Autodesk Inventor part; units mm, degrees
ref_plane "YZ Plane" through (0, 0, 0) normal (1, 0, 0) x (0, 1, 0)
ref_plane "XZ Plane" through (0, 0, 0) normal (0, 1, 0) x (-1, 0, 0)
ref_plane "XY Plane" through (0, 0, 0) normal (0, 0, 1) x (1, 0, 0)
sketch "Sketch1" plane through (0, 0, 0) normal (0, 1, 0) x (-1, 0, 0)
  line L0 (0, 0) -> (0, -15) construction
  line L1 (0, 0) -> (16, 0) construction
  arc A0 (-6, -15) -> (6, -15) centre (0, -15) ccw
  arc A1 (16, -6) -> (16, 6) centre (16, 0) ccw
  line L2 (-6, -15) -> (-6, -6)
  line L3 (0, -6) -> (-6, -6) construction
  line L4 (16, 6) -> (6, 6)
  line L5 (6, 6) -> (-6, 6) construction
  line L6 (-6, 6) -> (-6, -6) construction
  line L7 (16, -6) -> (6, -6)
  line L8 (6, -6) -> (0, -6) construction
  line L9 (6, -15) -> (6, -6)
  circle A2 centre (0, 0) radius 1.35
  line L10 (0, 0) -> (0, -12) construction
  line L11 (0, -12) -> (0, -15) construction
  line L12 (0, -15) -> (0, -18) construction
  line L13 (0, 0) -> (10, 0) construction
  line L14 (10, 0) -> (13, 0) construction
  line L15 (13, 0) -> (16, 0) construction
  line L16 (16, 0) -> (19, 0) construction
  circle A3 centre (19, 0) radius 0.75
  circle A4 centre (16, 0) radius 0.75
  circle A5 centre (13, 0) radius 0.75
  circle A6 centre (10, 0) radius 0.75
  circle A7 centre (0, -12) radius 0.75
  circle A8 centre (0, -15) radius 0.75
  circle A9 centre (0, -18) radius 0.75
  line L17 (6.8305, 0) -> (-5.2, 0)
  line L18 (0, -4.7373) -> (0, 4.2525)
  arc A10 (6, 15) -> (-6, 15) centre (0, 15) ccw
  line L19 (-6, 15) -> (-6, 6)
  line L20 (6, 15) -> (6, 6)
  circle A11 centre (0, 12) radius 0.75
  circle A12 centre (0, 15) radius 0.75
  circle A13 centre (0, 18) radius 0.75
  arc A14 (-16, 6) -> (-16, -6) centre (-16, 0) ccw
  line L21 (-16, 6) -> (-6, 6)
  line L22 (-16, -6) -> (-6, -6)
  circle A15 centre (-19, 0) radius 0.75
  circle A16 centre (-16, 0) radius 0.75
  circle A17 centre (-13, 0) radius 0.75
  circle A18 centre (-10, 0) radius 0.75
  dimension "d0" = 15
  dimension "d1" = 16
  dimension "d2" = 12
  dimension "d3" = 12
  dimension "d5" = 2.7
  dimension "d6" = 12
  dimension "d7" = 3
  dimension "d8" = 3
  dimension "d9" = 10
  dimension "d10" = 3
  dimension "d11" = 3
  dimension "d12" = 3
  dimension "d13" = 1.5
  dimension "d14" = 1.5
  dimension "d15" = 1.5
  dimension "d16" = 1.5
  dimension "d17" = 1.5
  dimension "d18" = 1.5
  dimension "d19" = 1.5
  dimension "d20" = 6
extrude "Extrusion1" add sketch "Sketch1" along normal blind 2.1
sketch "Sketch2" plane through (0, 2.1, 0) normal (0, 1, 0) x (1, 0, 0)
  circle A0 centre (0, 0) radius 3
  dimension "d23" = 6
extrude "Extrusion2" cut sketch "Sketch2" against normal blind 1.4
sketch "Sketch3" plane through (0, 0, 0) normal (0, -1, 0) x (1, 0, 0)
  circle A0 centre (0, 0) radius 1.35
  circle A1 centre (0, 0) radius 6
  dimension "d26" = 12
extrude "Extrusion3" add sketch "Sketch3" along normal blind 0.9
sketch "Sketch4" plane through (0, -0.9, 0) normal (0, -1, 0) x (1, 0, 0)
  circle A0 centre (0, 0) radius 1.35
  circle A1 centre (0, 0) radius 5
  dimension "d29" = 10
extrude "Extrusion4" add sketch "Sketch4" along normal blind 2.85
sketch "Sketch5" plane through (0, 0, 0) normal (0, -1, 0) x (1, 0, 0)
  line L0 (16, -6) -> (6, -6)
  arc A0 (-16, 6) -> (-16, -6) centre (-16, 0) ccw
  line L1 (16, -6) -> (-16, -6)
  line L2 (6, 6) -> (16, 6)
  line L3 (16, 6) -> (-16, 6)
  circle A1 centre (-16, 0) radius 0.75
  arc A2 (-16, 6) -> (-16, -6) centre (-16, 0) ccw
  circle A3 centre (16, 0) radius 0.75
  arc A4 (16, -6) -> (16, 6) centre (16, 0) ccw
  circle A5 centre (-10, 0) radius 0.75
  circle A6 centre (-10, 0) radius 0.75
  circle A7 centre (-13, 0) radius 0.75
  circle A8 centre (-13, 0) radius 0.75
  circle A9 centre (-19, 0) radius 0.75
  circle A10 centre (-19, 0) radius 0.75
  circle A11 centre (-16, 0) radius 0.75
  circle A12 centre (10, 0) radius 0.75
  circle A13 centre (10, 0) radius 0.75
  circle A14 centre (13, 0) radius 0.75
  circle A15 centre (13, 0) radius 0.75
  circle A16 centre (16, 0) radius 0.75
  circle A17 centre (19, 0) radius 0.75
  circle A18 centre (19, 0) radius 0.75
  point P0 (0, 0)
extrude "Extrusion5" add sketch "Sketch5" along normal blind 0.9
sketch "Sketch6" plane through (0, -0.9, 0) normal (0, -1, 0) x (1, 0, 0)
  circle A0 centre (0, 0) radius 1.35
  circle A1 centre (0, 0) radius 1.35
extrude "Extrusion6" cut sketch "Sketch6" against normal blind 0.9
sketch "Sketch7" plane through (0, -3.75, 0) normal (0, -1, 0) x (1, 0, 0)
  circle A0 centre (0, 0) radius 1.35
  circle A1 centre (0, 0) radius 2.75
  dimension "d36" = 5.5
extrude "Extrusion7" cut sketch "Sketch7" against normal blind 3 contours A0 | A1
properties part number "MMAE 232 CAD Assignment 2 Servo Horn 3-Nicholas Skiba"
Check sheet for the modelled part. Datum: model origin and axes. Units: mm. A direction names the side the tool comes from. Give positions to 0.01 mm unless a question says otherwise; leave off trailing zeros. Write each loop counter-clockwise with the first axis right and the second up, starting at its lowest first coordinate (ties: lowest second). Pieces come first, ordered by that corner, then holes. Notation, with made-up numbers: (24.5, -4.5) -> (64.5, -4.5) arc R18 ccw to (64.5, 30.5) -> close; hole circle Ø11 at (87.5, -29). An arc over 180 degrees is marked (long way). One line per item, written item: value. Start each with the question number.
Item 1: Section check A-A on x = 13. Record the cut outline in (y, z).
Item 2: Tool access check on faces 5 (the flat face through (0, 0, 14)), 6 (the flat face through (-6, 1, 11)), 7 (the flat face through (6, 1, -11)), 8 (the flat face through (6, 1, 11)), 9 (the flat face through (0, 0, -13)). Record the directions out of +Z, -Z, +X, -X, +Y, -Y that give a thin tool (end or side, any length) a straight path to the whole face; none if there is none.
Item 3: Gauge pin test, flat ends, axial feed: pin 1 (1 mm diameter, centred on x = -2.5, z = 1.5, fed in from +Y); pin 2 (1.7 mm diameter, centred on x = -16, z = 0, fed in from -Y); pin 3 (2.5 mm diameter, centred on x = -1.5, y = 1, fed in from +Z); pin 4 (1.5 mm diameter, centred on x = 4.5, z = -10, fed in from -Y). Record the tip position at first contact, or that the pin passes through.
Item 4: Material ranges on probe 1 along Z at (x, y) = (-13, -0.45); probe 2 along Z at (x, y) = (0, -0.5); probe 3 along Y at (x, z) = (19, -2), recorded low to high. Write a range as from..to.
Item 5: Section check B-B on z = 18. Record the cut outline in (x, y).
Item 6: Section check C-C on y = -3.2. Record the cut outline in (x, z).
Item 7: Draft check along Z on faces 1 (the cylindrical face through (0.098, 1.035, 11.256)), 2 (the cylindrical face through (22, 1, 0)), 3 (the cylindrical face through (0, 1, 21)), 4 (the cylindrical face through (-3, 1, 0)). Enter one of: +Z half, -Z half, draft (parallel to the pull), parting line (faces both ways), or undercut.
Item 8: Section check D-D on z = -3.5. Record the cut outline in (x, y).
Results list:
1. outline: (-0.9, -6) -> (2.1, -6) -> (2.1, -0.75) -> (-0.9, -0.75) -> close; (-0.9, 0.75) -> (2.1, 0.75) -> (2.1, 6) -> (-0.9, 6) -> close
2. face 5: +Z, +X, -X, -Y
2. face 6: +Z, -X, +Y, -Y
2. face 7: -Z, +X, +Y, -Y
2. face 8: +Z, +X, +Y, -Y
2. face 9: -Z, +X, -X, -Y
3. pin 1: y = 2.1
3. pin 2: y = -0.9
3. pin 3: z = 20.99
3. pin 4: y = 0
4. probe 1: -6..-0.75, 0.75..6
4. probe 2: -6..-1.35, 1.35..6
4. probe 3: -0.9..2.1
5. outline: (-5.2, 0) -> (-0.75, 0) -> (-0.75, 2.1) -> (-5.2, 2.1) -> close; (0.75, 0) -> (5.2, 0) -> (5.2, 2.1) -> (0.75, 2.1) -> close
6. outline: circle Ø10 at (0, 0); hole circle Ø5.5 at (0, 0)
7. face 1: undercut
7. face 2: parting line
7. face 3: +Z half
7. face 4: undercut
8. outline: (-20.87, -0.9) -> (-3.57, -0.9) -> (-3.57, -3.75) -> (3.57, -3.75) -> (3.57, -0.9) -> (20.87, -0.9) -> (20.87, 2.1) -> (-20.87, 2.1) -> close
